Verification items for the finished model (mm, model axes). Face numbers are marked on the shaded views. A direction names the side the tool comes from. Round coordinates to 2 decimals unless told otherwise and drop trailing zeros. Write each loop counter-clockwise with the first axis right and the second up, starting at its lowest first coordinate (ties: lowest second). Pieces come first, ordered by that corner, then holes.
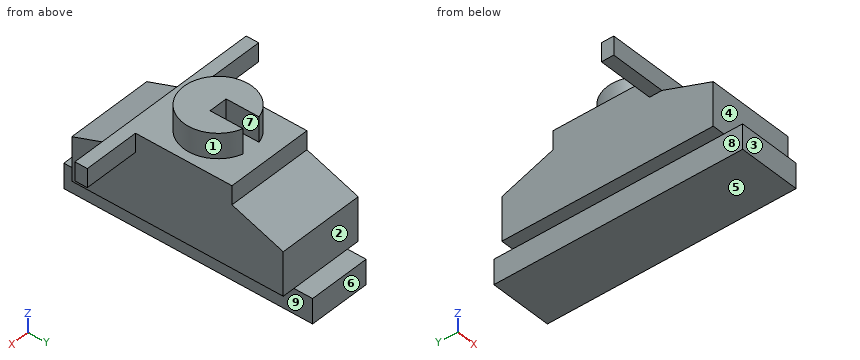
from build123d import *

# Parameters (mm, degrees)
SKETCH_1_W           = 10
SKETCH_1_H           = 40
EXTRUDE_1_DEPTH      = 4
EXTRUDE_2_DEPTH      = 7
EXTRUDE_2_DEPTH_BACK = 7
SKETCH_4_W           = 32
SKETCH_4_H           = 3
EXTRUDE_3_DEPTH      = 2
SKETCH_5_R           = 5.5
EXTRUDE_4_DEPTH      = 4
SKETCH_6_W           = 3
SKETCH_6_H           = 5.5
CUT_EXTRUDE_1_DEPTH  = 4


with BuildPart() as part:
    # Эскиз1 → Бобышка-Вытянуть1 (new body)
    with BuildSketch(Plane.XY):
        Rectangle(SKETCH_1_W, SKETCH_1_H)
    extrude(amount=EXTRUDE_1_DEPTH)

    # Эскиз3 → Бобышка-Вытянуть2 (add, two sides: drawn at the far end of the back side and taken through both)
    with BuildSketch(Plane(origin=(0, 0, 0), x_dir=(0, 0, -1), z_dir=(1, 0, 0)).offset(-EXTRUDE_2_DEPTH_BACK)):
        Polygon((-17, -8.757567742), (-17, 8.757567742), (-14, 8.757567742), (-11, 17), (-4, 17), (-4, -17), (-11, -17), (-14, -8.757567742), align=None)
    extrude(amount=EXTRUDE_2_DEPTH + EXTRUDE_2_DEPTH_BACK)

    # Эскиз4 → Бобышка-Вытянуть3 (add)
    with BuildSketch(Plane.XZ.offset(8.757567742)):
        with Locations((0, 15.5)):
            Rectangle(SKETCH_4_W, SKETCH_4_H)
    extrude(amount=-EXTRUDE_3_DEPTH)

    # Эскиз5 → Бобышка-Вытянуть4 (add)
    with BuildSketch(Plane.XY.offset(17)):
        with Locations(Location((0, 0.5, 0), (0, 0, 180))):
            Circle(SKETCH_5_R)
    extrude(amount=EXTRUDE_4_DEPTH)

    # Эскиз6 → Вырез-Вытянуть1 (cut)
    with BuildSketch(Plane.XY.offset(21)):
        with Locations((0, 3.25)):
            Rectangle(SKETCH_6_W, SKETCH_6_H)
    extrude(amount=-CUT_EXTRUDE_1_DEPTH, mode=Mode.SUBTRACT)


solid = part.part
Q1. Sectioned sample at B-B (x = 0). Enter the section's corners in (y, z).
Recorded:
outline: (-20, 0) - (20, 0) - (20, 4) - (17, 4) - (17, 11) - (8.76, 14) - (8.76, 17) - (0.5, 17) - (0.5, 21) - (-5, 21) - (-5, 17) - (-8.76, 17) - (-8.76, 14) - (-17, 11) - (-17, 4) - (-20, 4) - close
Q2. Sectioned sample at A-A (y = 7). Enter the section's corners in (x, z).
Recorded:
outline: (-7, 4) - (-5, 4) - (-5, 0) - (5, 0) - (5, 4) - (7, 4) - (7, 17) - (-7, 17) - close
Q3. Depth check by flat-ended pin: P1, Ø1, axis at x = -6, y = 0.5, coming from the -Z side; P2, Ø10.5, axis at y = 1.5, z = 9, coming from the -X side; P3, Ø2, axis at x = -1, z = 6, coming from the -Y side. Enter the tip coordinate at first touch or a pass-through.
Recorded:
P1: stops at z = 4
P2: stops at x = -7
P3: stops at y = -17
Q4. Sectioned sample at D-D (y = -8). Enter the section's corners in (x, z), plus the area to 3 significant figures.
Recorded:
outline: (-16, 14) - (-7, 14) - (-7, 4) - (-5, 4) - (-5, 0) - (5, 0) - (5, 4) - (7, 4) - (7, 14) - (16, 14) - (16, 17) - (-16, 17) - close
area: 276 mm2
Q5. Material ranges on line 1 along X through (y, z) = (6.5, 8.5); line 2 along X through (y, z) = (2, 1.5); line 3 along Y through (x, z) = (-2, 4.75), recorded low to high.
Recorded:
line 1: x = -7 to 7
line 2: x = -5 to 5
line 3: y = -17 to 17
Q6. Tool access check on the marked faces 1, 2, 3, 4 and 5. Record the directions out of +Z, -Z, +X, -X, +Y, -Y that give a thin tool (end or side, any length) a straight path to the whole face; none if there is none.
Recorded:
face 1: +Z
face 2: +Z, +X, -X, +Y
face 3: +Z, -Z, +X, -X, -Y
face 4: +Z, +X, -X, -Y
face 5: -Z, +X, -X, +Y, -Y
Q7. Sectioned sample at C-C (z = 2.5). Enter the section's corners in (x, y).
Recorded:
outline: (-5, -20) - (5, -20) - (5, 20) - (-5, 20) - close
Q8. Release check for a two-part mould opening along X. For the marked faces 6, 7, 8 and 9 record: released by +X, released by -X, zero draft, split by the parting line, or undercut.
Recorded:
face 6: zero draft
face 7: undercut
face 8: released by -X
face 9: released by +X
